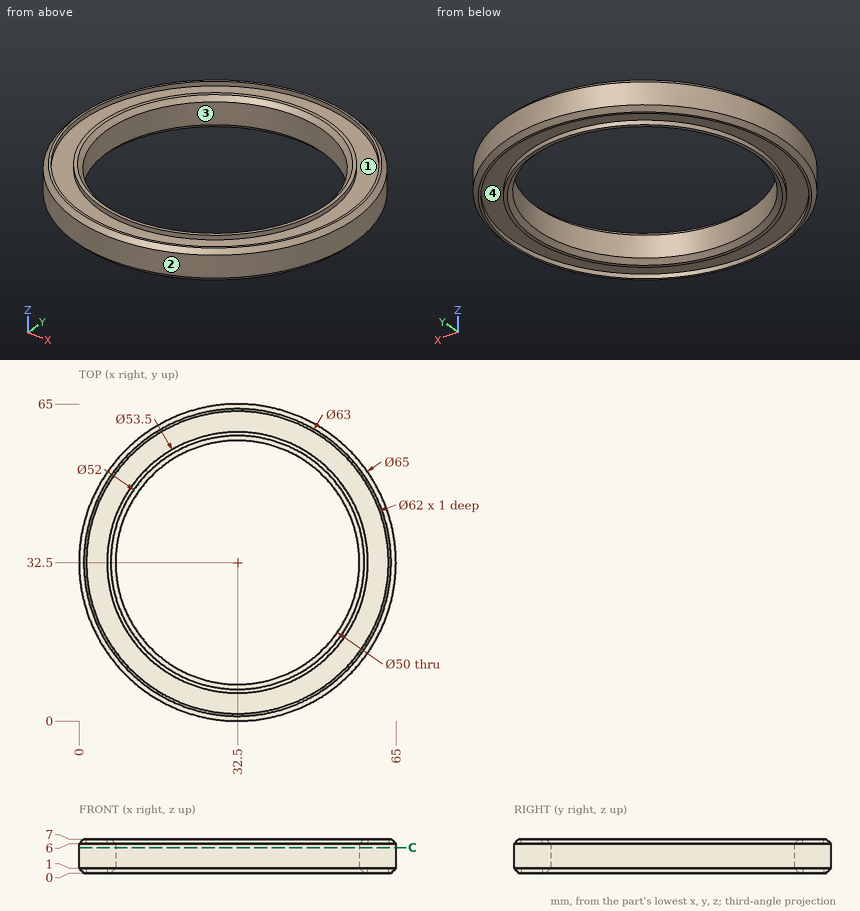
Verification items for this drawing (mm, ordinates from the low corner). A direction names the side the tool comes from. Round coordinates to 2 decimals unless told otherwise and drop trailing zeros. Loops run counter-clockwise (first coordinate to the right, second up) from the corner with the lowest first, then second, coordinate; pieces in that order, holes last. Notation, with made-up numbers: M 48.25,-2.75 L 67.25,-2.75 A11 ccw 67.25,1.25 Z; hole C 22,72.25 d4. An arc over 180 degrees is marked long. Answer as a JSON object with one key per item and string values.
1. Scan lines: line 1 (Y direction, x = 32.5, z = 4.8); line 2 (Z direction, x = 14, y = 7); line 3 (Y direction, x = 32.5, z = 6.55). Record each from-to range of solid material in increasing order.
Reply:
{"line 1": "y = 0 to 7.5, 57.5 to 65", "line 2": "z = 0 to 7", "line 3": "y = 0.55 to 1.5, 5.75 to 6.95, 58.05 to 59.25, 63.5 to 64.45"}
2. Section check C-C (z = 5.25). Record the boundary of the cut face in (x, y), plus the area to 3 significant figures.
Reply:
{"outline": "C 32.5,32.5 d65; hole C 32.5,32.5 d50", "area": "1,350 mm²"}
3. Access from +Z, -Z, +X, -X, +Y, -Y to the whole of each face (thin tool, end or side, straight path). Record for the marked faces 3 and 4.
Reply:
{"face 3": "+Z, -Z", "face 4": "-Z"}
4. Gauge pin test, flat ends, axial feed: P1, Ø2, axis at x = 48.5, z = 1.5, coming from the -Y side; P2, Ø2, axis at x = 56, z = 2, coming from the -Y side. Record the tip position at first contact, or that the pin passes through.
Reply:
{"P1": "stops at y = 3.67", "P2": "stops at y = 9.05"}
5. Mould release check, pull along X, two halves, no side actions. Record for the marked faces 1 and 2: pulls with the +X half, pulls with the -X half, needs draft (parallel to the pull), parting line crosses it, or undercut.
Reply:
{"face 1": "undercut", "face 2": "parting line crosses it"}
